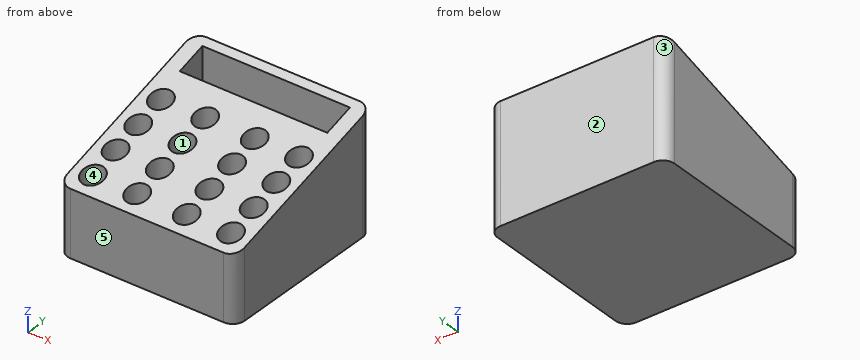
from build123d import *

# Parameters (mm, degrees)
F0_W     = 76.2
F0_H     = 76.2
F1_DEPTH = 50.8
F2_R     = 4.7625
F2_W     = 63.5
F2_H     = 12.7
F3_DEPTH = 44.45
F5_DEPTH = 76.2
F6_R     = 5.08


with BuildPart() as f1:
    # F0 (on Top) → F1 (new body)
    with BuildSketch(Plane.XY):
        with Locations((-4.885403, 0.97207)):
            Rectangle(F0_W, F0_H)
    extrude(amount=F1_DEPTH)

    # F2 (on face) → F3 (cut)
    with BuildSketch(Plane.XY.offset(50.8)):
        with Locations((-34.603403, 9.35407)):
            Circle(F2_R)
        with Locations((-15.553403, 9.35407)):
            Circle(F2_R)
        with Locations((-34.603403, -3.34593)):
            Circle(F2_R)
        with Locations((-34.603403, -16.04593)):
            Circle(F2_R)
        with Locations((-34.603403, -28.74593)):
            Circle(F2_R)
        with Locations((-15.553403, -3.34593)):
            Circle(F2_R)
        with Locations((-15.553403, -16.04593)):
            Circle(F2_R)
        with Locations((-15.553403, -28.74593)):
            Circle(F2_R)
        with Locations((5.782597, 9.35407)):
            Circle(F2_R)
        with Locations((5.782597, -3.34593)):
            Circle(F2_R)
        with Locations((5.782597, -16.04593)):
            Circle(F2_R)
        with Locations((5.782597, -28.74593)):
            Circle(F2_R)
        with Locations((24.832597, 9.35407)):
            Circle(F2_R)
        with Locations((24.832597, -3.34593)):
            Circle(F2_R)
        with Locations((24.832597, -16.04593)):
            Circle(F2_R)
        with Locations((24.832597, -28.74593)):
            Circle(F2_R)
        with Locations((-4.885403, 28.906011)):
            Rectangle(F2_W, F2_H)
    extrude(amount=-F3_DEPTH, mode=Mode.SUBTRACT)

    # F4 (on face) → F5 (cut)
    with BuildSketch(Plane(origin=(-42.985403, 0, 0), x_dir=(0, -1, 0), z_dir=(-1, 0, 0))):
        Polygon((37.12793, 50.8), (-39.07207, 50.8), (37.12793, 28.298467), align=None)
    extrude(amount=-F5_DEPTH, mode=Mode.SUBTRACT)

    # F6
    f6_edges = [f1.edges().sort_by_distance(p)[0] for p in [
        (33.214597, -37.12793, 14.149234),
        (-42.985403, -37.12793, 14.149234),
        (33.214597, 39.07207, 25.4),
        (-42.985403, 39.07207, 25.4),
    ]]
    fillet(f6_edges, radius=F6_R)


solid = f1.part
Here's how the part is built. I have some questions about the finished solid (model axes, mm). Face numbers are marked on the shaded views. A direction names the side the tool comes from. Give positions to 0.01 mm unless a question says otherwise; leave off trailing zeros. Order: outer loops, then holes, each group sorted by start corner. A loop starts at its lowest first (then second) coordinate and runs counter-clockwise, first axis right, second up. Notation, with made-up numbers: M 45.5,1.25 L 70.5,1.25 A20 ccw 70.5,35.25 Z; hole C -5,51 d11. An arc over 180 degrees is marked long. Answer as a JSON object with one key per item and string values. Group by question number.
1) We'd pull the mould along X, two halves only. Please class the marked faces 3, 4 and 5: pulls with the +X half, pulls with the -X half, needs draft (parallel to the pull), parting line crosses it, or undercut.
2) I'm going to push flat-ended pins straight in: pin 1 Ø10.5 at (x, y) = (26.5, 11.5) entering from +Z; pin 2 Ø10.5 at (x, y) = (-17, -30) entering from +Z; pin 3 Ø7.5 at (x, y) = (24.83, -16.05) entering from -Z; pin 4 Ø10.5 at (x, y) = (-34, 11) entering from +Z. Where does each tip first touch, or does it pass through?
3) Suppose I cut it at B-B, the plane y = 30. Write out the boundary of the cut face in (x, z), plus the area to 3 significant figures.
4) Suppose I cut it at D-D, the plane z = 25. Count the separate pieces of the cut face and the enclosed holes in it, plus the area to 3 significant figures.
5) Please list where these lines run through material, in increasing order: L1, parallel to X at y = -28.5, z = 20; L2, parallel to X at y = -3, z = 38; L3, parallel to Y at x = 13, z = 10.5. Write a range as [from, to].
6) Suppose I cut it at A-A, the plane z = 41. Write out the boundary of the cut face in (x, y) (1 decimal), plus the area to 3 significant figures.
7) On a 3-axis mill with a long thin cutter (end or side, diameter ignored), from which of +Z, -Z, +X, -X, +Y, -Y can I reach the whole of each face in a straight line? I mean the marked faces 1 and 2. Say none if no direction works.
8) Suppose I cut it at C-C, the plane x = -5.5. Write out the boundary of the cut face in (y, z), plus the area to 3 significant figures.
Results found:
{
 "1": {"face 3": "pulls with the -X half", "face 4": "undercut", "face 5": "needs draft"},
 "2": {"pin 1": "z = 44.21", "pin 2": "z = 31.9", "pin 3": "z = 0", "pin 4": "z = 44.06"},
 "3": {"outline": "M -42.99,0 L 33.21,0 L 33.21,48.12 L 26.86,48.12 L 26.86,6.35 L -36.64,6.35 L -36.64,48.12 L -42.99,48.12 Z", "area": "1,010 mm²"},
 "4": {"separate pieces": "1", "enclosed holes": "17", "area": "3,840 mm²"},
 "5": {"L1": "[-42.99, -39.36], [-29.85, -20.31], [-10.8, 1.03], [10.54, 20.08], [29.59, 33.21]", "L2": "[-42.99, -39.35], [-29.85, -20.3], [-10.8, 1.03], [10.53, 20.08], [29.58, 33.21]", "L3": "[-37.13, 22.56], [35.26, 39.07]"},
 "6": {"outline": "M -43,5.9 L -37.9,5.9 A4.8 cw long -31.3,5.9 L -18.8,5.9 A4.8 cw long -12.3,5.9 L 2.5,5.9 A4.8 cw long 9,5.9 L 21.6,5.9 A4.8 cw long 28.1,5.9 L 33.2,5.9 L 33.2,34 A5.1 ccw 28.1,39.1 L -37.9,39.1 A5.1 ccw -43,34 Z; hole M -36.6,22.6 L 26.9,22.6 L 26.9,35.3 L -36.6,35.3 Z", "area": "1,450 mm²"},
 "7": {"face 1": "+Z", "face 2": "+Z, -Z, +X, -X, +Y"},
 "8": {"outline": "M -37.13,0 L 39.07,0 L 39.07,50.8 L 35.26,49.67 L 35.26,6.35 L 22.56,6.35 L 22.56,45.92 L -37.13,28.3 Z", "area": "2,490 mm²"}
}
